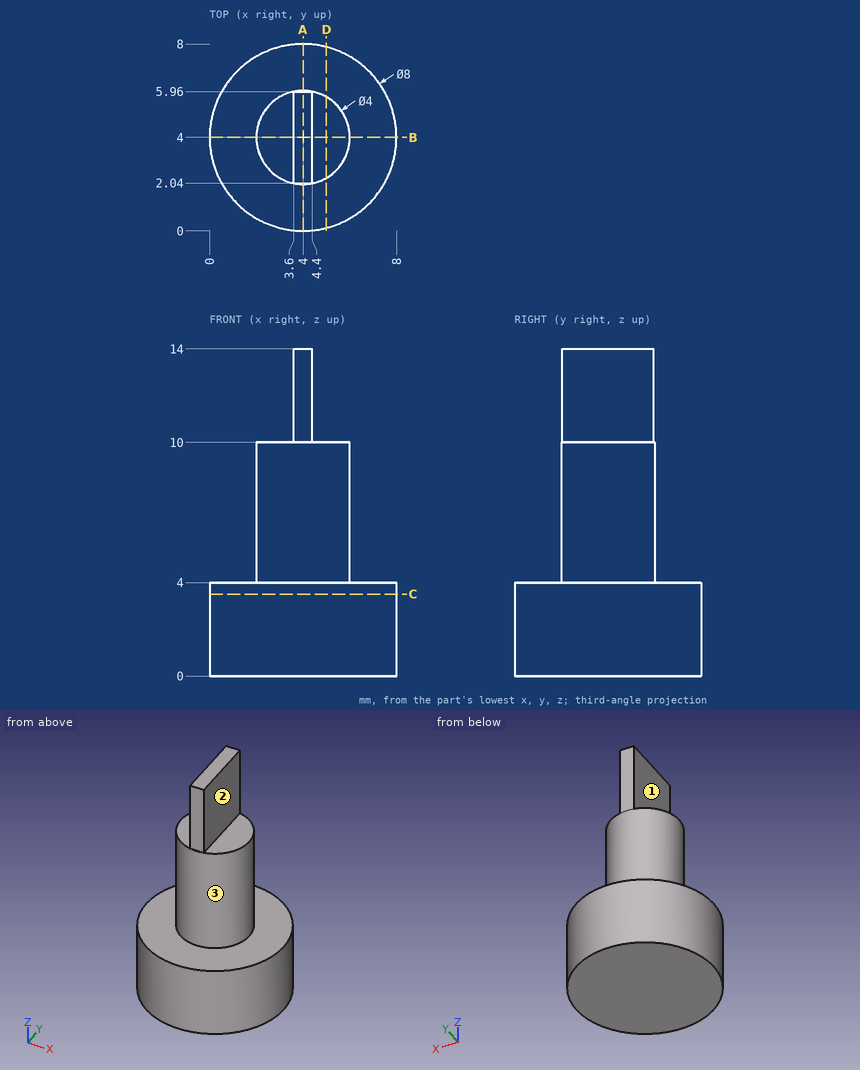
Here's the drawing with two shaded views (mm, measured from the low corner). I have some questions. A direction names the side the tool comes from. Give positions to 0.01 mm unless a question says otherwise; leave off trailing zeros. Write each loop counter-clockwise with the first axis right and the second up, starting at its lowest first coordinate (ties: lowest second). Pieces come first, ordered by that corner, then holes. Notation, with made-up numbers: (13.5, 58) - (62.5, 58) arc R23 cw to (62.5, 75) - close; hole circle Ø3 at (-31, -10.75). An arc over 180 degrees is marked (long way). One line per item, written item: value. Start each with the question number.
Item 1: Please list where these lines run through material, in increasing order: line 1 (X direction, y = 2.5, z = 11.5); line 2 (Z direction, x = 2.25, y = 7.5); line 3 (Z direction, x = 4.5, y = 2.5). Write a range as from..to.
Item 2: I'm going to push flat-ended pins straight in: pin 1 (4.5 mm diameter, centred on y = 4.5, z = 12, fed in from -X); pin 2 (1.5 mm diameter, centred on x = 6.5, z = 4, fed in from -Y); pin 3 (1 mm diameter, centred on y = 3, z = 8.5, fed in from -X). Where does each tip first touch, or does it pass through?
Item 3: Imagine slicing it at D-D, the plane x = 5. List the corners of the cut face in (y, z) for me.
Item 4: Imagine slicing it at A-A, the plane x = 4. List the corners of the cut face in (y, z) for me.
Item 5: Imagine slicing it at B-B, the plane y = 4. List the corners of the cut face in (x, z) for me.
Item 6: Which directions (+Z, -Z, +X, -X, +Y, -Y) give clear straight access to the entire face, cutting with the end or side of a thin tool? Please do the marked faces 1, 2 and 3.
Item 7: Imagine slicing it at C-C, the plane z = 3.5. List the corners of the cut face in (x, y) for me.
Geometry says:
1. line 1: 3.6..4.4
1. line 2: 0..4
1. line 3: 0..10
2. pin 1: x = 2
2. pin 2: y = 0.4
2. pin 3: x = 2.06
3. outline: (0.13, 0) - (7.87, 0) - (7.87, 4) - (5.73, 4) - (5.73, 10) - (2.27, 10) - (2.27, 4) - (0.13, 4) - close
4. outline: (0, 0) - (8, 0) - (8, 4) - (6, 4) - (6, 10) - (5.96, 10) - (5.96, 14) - (2.04, 14) - (2.04, 10) - (2, 10) - (2, 4) - (0, 4) - close
5. outline: (0, 0) - (8, 0) - (8, 4) - (6, 4) - (6, 10) - (4.4, 10) - (4.4, 14) - (3.6, 14) - (3.6, 10) - (2, 10) - (2, 4) - (0, 4) - close
6. face 1: +Z, -X, +Y, -Y
6. face 2: +Z, +X, +Y, -Y
6. face 3: +Z
7. outline: circle Ø8 at (4, 4)
